Part model, mm, in its own coordinate system. A direction names the side the tool comes from. Coordinates: 2 decimals unless noted, no trailing zeros. Order: outer loops, then holes, each group sorted by start corner. A loop starts at its lowest first (then second) coordinate and runs counter-clockwise, first axis right, second up. Notation, with made-up numbers: (68, -8.75) - (127, -8.75) arc R20 cw to (127, 25.25) - close; hole circle Ø1 at (56.5, 74.5). An arc over 180 degrees is marked (long way). Use a Markdown table: item, result. Add a question column.
1) Wall check: L1, parallel to Z at x = 50, y = 1.6; L2, parallel to X at y = 14, z = 18; L3, parallel to Y at x = 53, z = 2. Give the ranges that are in metal, low to high. Write a range as [from, to].
2) Saw through at B-B on z = 12.5. List the corners of the cut face in (x, y), then the cut area to 3 significant figures.
3) Saw through at A-A on y = 5.5. List the corners of the cut face in (x, z).
4) Tool access for faces 4 (the face through (39, 0, 12)), 5 (the face through (17, 1, 12.6)), 6 (the face through (78, 12, 12)): list every direction of +Z, -Z, +X, -X, +Y, -Y with a clear straight run to the whole face (end or side of a thin tool).
5) Saw through at C-C on x = 20. List the corners of the cut face in (y, z).
6) Drop flat-ended pins along their axis: P1, Ø8, axis at x = 28.5, z = 9, coming from the +Y side; P2, Ø12, axis at x = 67, z = 13, coming from the +Y side; P3, Ø8, axis at x = 50, z = 12.5, coming from the +Y side. Give the stop position or say it passes through.
7) Saw through at D-D on z = 19.5. List the corners of the cut face in (x, y).
8) Two-plate mould, pull along X, no slides. Class faces 1 (the face through (80, 12, 12)), 2 (the face through (0, 18, 12)), 3 (the face through (40.53, 27.81, 12.32)): +X half, -X half, draft (parallel to the pull), parting line (faces both ways), or undercut.
```python
from build123d import *

# Parameters (mm, degrees)
BOSS_EXTRUDE1_DEPTH = 25
SKETCH4_R           = 3
CUT_EXTRUDE1_DEPTH  = 17


with BuildPart() as part:
    # Sketch3 → Boss-Extrude1 (new body)
    with BuildSketch(Plane.XY):
        Polygon((0, 35.853266996), (0, 0), (80, 0), (80, 23.970502896), align=None)
        Polygon((2, 33.534255745), (2, 2), (78, 2), (78, 22.24562985), align=None, mode=Mode.SUBTRACT)
    extrude(amount=BOSS_EXTRUDE1_DEPTH)

    # Sketch4 → Cut-Extrude1 (cut)
    with BuildSketch(Plane.XZ):
        with Locations((20, 12.5)):
            Circle(SKETCH4_R)
        with Locations((50, 12.5)):
            Circle(SKETCH4_R)
    extrude(amount=-CUT_EXTRUDE1_DEPTH, mode=Mode.SUBTRACT)


solid = part.part
```
Results are:
| question | item | result |
|---|---|---|
| 1 | L1 | [0, 9.5], [15.5, 25] |
| 1 | L2 | [0, 2], [78, 80] |
| 1 | L3 | [0, 2], [25.96, 27.98] |
| 2 | outline | (0, 0) - (17, 0) - (17, 2) - (2, 2) - (2, 33.53) - (78, 22.25) - (78, 2) - (53, 2) - (53, 0) - (80, 0) - (80, 23.97) - (0, 35.85) - close; (23, 0) - (47, 0) - (47, 2) - (23, 2) - close |
| 2 | area | 401 mm2 |
| 3 | outline | (0, 0) - (2, 0) - (2, 25) - (0, 25) - close; (78, 0) - (80, 0) - (80, 25) - (78, 25) - close |
| 4 | face 4 | +Z, -Z, +X, -X, -Y |
| 4 | face 5 | -Y |
| 4 | face 6 | +Z, -Z |
| 5 | outline | (0, 0) - (2, 0) - (2, 9.5) - (0, 9.5) - close; (0, 15.5) - (2, 15.5) - (2, 25) - (0, 25) - close; (30.86, 0) - (32.88, 0) - (32.88, 25) - (30.86, 25) - close |
| 6 | P1 | y = 32.21 |
| 6 | P2 | y = 26.79 |
| 6 | P3 | y = 29.02 |
| 7 | outline | (0, 0) - (80, 0) - (80, 23.97) - (0, 35.85) - close; hole (2, 2) - (78, 2) - (78, 22.25) - (2, 33.53) - close |
| 8 | face 1 | +X half |
| 8 | face 2 | -X half |
| 8 | face 3 | undercut |
